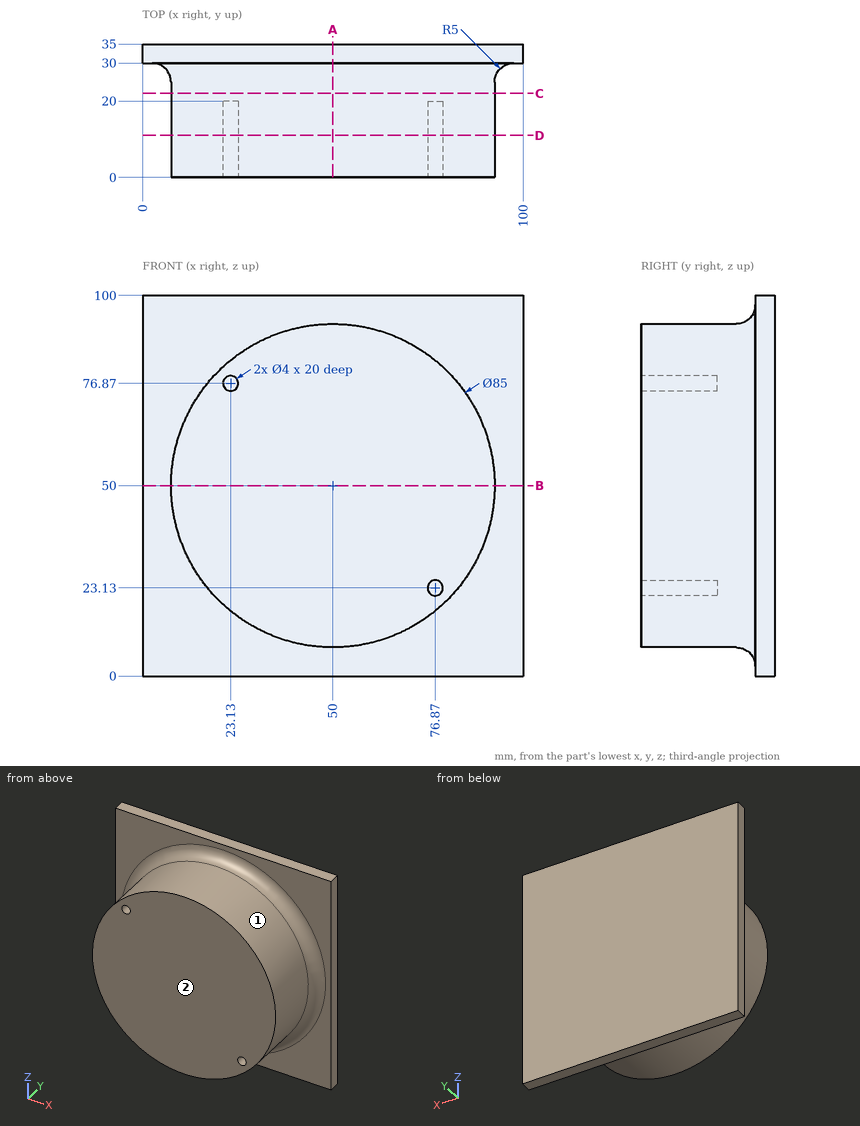
Can you work these out from the drawing? Everything is in mm from the part's minimum corner. A direction names the side the tool comes from. Give positions to 0.01 mm unless a question says otherwise; leave off trailing zeros. Order: outer loops, then holes, each group sorted by start corner. A loop starts at its lowest first (then second) coordinate and runs counter-clockwise, first axis right, second up. Notation, with made-up numbers: M 21.5,11.5 L 54.5,11.5 A13 cw 54.5,32.5 Z; hole C -39.75,-15 d11. An arc over 180 degrees is marked long. Use a Markdown table: item, result. Add a question column.
Item 1: Suppose I cut it at C-C (y = 22). List the corners of the cut face in (x, z) for me.
Item 2: If I drill on L1, parallel to Z at x = 49, y = 11; L2, parallel to Y at x = 24, z = 8.5; L3, parallel to X at y = 2, z = 23.5, over which ranges is the centre line in solid material (lowest first)? Write a range as [from, to].
Item 3: For the marked faces 1 and 2, which set-ups out of +Z, -Z, +X, -X, +Y, -Y let a thin tool reach every point of the face, with its end or its side?
Item 4: Suppose I cut it at B-B (z = 50). List the corners of the cut face in (x, y) for me, then the cut area to 3 significant figures.
Item 5: Suppose I cut it at D-D (y = 11). List the corners of the cut face in (x, z) for me.
Item 6: Suppose I cut it at A-A (x = 50). List the corners of the cut face in (y, z) for me.
Item 7: Will these pins go through, and if not, where does the flat tip stop? pin 1 (4 mm diameter, centred on y = 27, z = 67.5, fed in from +X); pin 2 (4 mm diameter, centred on x = 28, y = 10, fed in from -Z); pin 3 (3 mm diameter, centred on x = 23, z = 76.5, fed in from -Y).
Answer sheet:
| question | item | result |
|---|---|---|
| 1 | outline | C 50,50 d85 |
| 2 | L1 | z = [7.51, 92.49] |
| 2 | L2 | y = [30, 35] |
| 2 | L3 | x = [16.77, 74.9], [78.84, 83.23] |
| 3 | face 1 | -Y |
| 3 | face 2 | +Z, -Z, +X, -X, -Y |
| 4 | outline | M 0,30 L 2.5,30 A5 cw 7.5,25 L 7.5,0 L 92.5,0 L 92.5,25 A5 cw 97.5,30 L 100,30 L 100,35 L 0,35 Z |
| 4 | area | 3,060 mm² |
| 5 | outline | C 50,50 d85; hole C 23.13,76.87 d4; hole C 76.87,23.13 d4 |
| 6 | outline | M 0,7.5 L 25,7.5 A5 cw 30,2.5 L 30,0 L 35,0 L 35,100 L 30,100 L 30,97.5 A5 cw 25,92.5 L 0,92.5 Z |
| 7 | pin 1 | stops at x = 91.04 |
| 7 | pin 2 | stops at z = 12.5 |
| 7 | pin 3 | stops at y = 20 |
